Source: CAD feature listing. Evaluate the final solid. Frame: model axes, mm. A direction names the side the tool comes from. Give positions to 0.01 mm unless a question says otherwise; leave off trailing zeros. Loops run counter-clockwise (first coordinate to the right, second up) from the corner with the lowest first, then second, coordinate; pieces in that order, holes last.
from build123d import *

# Parameters (mm, degrees)
SKETCH1_R               = 25
BOSS_EXTRUDE1_DEPTH     = 10
SKETCH2_R               = 17.5
BOSS_EXTRUDE2_DEPTH     = 18
BOSS_EXTRUDE3_DEPTH     = 28
BOSS_EXTRUDE6_DEPTH     = 12
SKETCH5_W               = 12
SKETCH5_H               = 30
CUT_EXTRUDE3_DEPTH      = 35.5
CUT_EXTRUDE3_DEPTH_BACK = 35.5


with BuildPart() as part:
    # Sketch1 → Boss-Extrude1 (new body)
    with BuildSketch(Plane(origin=(0, 0, 0), x_dir=(1, 0, 0), z_dir=(0, 1, 0))):
        Circle(SKETCH1_R)
    extrude(amount=BOSS_EXTRUDE1_DEPTH)

    # Sketch2 → Boss-Extrude2 (add)
    with BuildSketch(Plane(origin=(0, 10, 0), x_dir=(1, 0, 0), z_dir=(0, 1, 0))):
        Circle(SKETCH2_R)
    extrude(amount=BOSS_EXTRUDE2_DEPTH)

    # Sketch3 → Boss-Extrude3 (add)
    with BuildSketch(Plane(origin=(0, 28, 0), x_dir=(1, 0, 0), z_dir=(0, 1, 0))):
        with BuildLine():
            Line((-15.564382416, -8), (15.564382416, -8))
            ThreePointArc((15.564382416, -8), (17.5, 0), (15.564382416, 8))
            Line((15.564382416, 8), (-15.564382416, 8))
            ThreePointArc((-15.564382416, 8), (-17.5, 0), (-15.564382416, -8))
        make_face()
    extrude(amount=BOSS_EXTRUDE3_DEPTH)

    # Sketch4 → Boss-Extrude6 (add, symmetric)
    with BuildSketch(Plane(origin=(0, 0, 0), x_dir=(0, 0, -1), z_dir=(1, 0, 0))):
        Polygon((34.5, 0), (34.5, 7), (25, 28), (-25, 28), (-34.5, 7), (-34.5, 0), align=None)
    extrude(amount=BOSS_EXTRUDE6_DEPTH, both=True)

    # Sketch5 → Cut-Extrude3 (cut, two sides)
    with BuildSketch(Plane.XY) as cut_extrude3_sk:
        with Locations((0, 29)):
            Rectangle(SKETCH5_W, SKETCH5_H)
    extrude(amount=CUT_EXTRUDE3_DEPTH, mode=Mode.SUBTRACT)
    extrude(cut_extrude3_sk.sketch, amount=-CUT_EXTRUDE3_DEPTH_BACK, mode=Mode.SUBTRACT)


solid = part.part
1) Cut plane C-C (z = 24). Return loops of the section in (x, y).
Checks:
outline: (-12, 0) - (12, 0) - (12, 28) - (6, 28) - (6, 14) - (-6, 14) - (-6, 28) - (-12, 28) - close
2) Cut plane D-D (y = 4). Return loops of the section in (x, z).
Checks:
outline: (-12, -34.5) - (12, -34.5) - (12, -21.93) arc R25 ccw to (12, 21.93) - (12, 34.5) - (-12, 34.5) - (-12, 21.93) arc R25 ccw to (-12, -21.93) - close
3) Contact query for flat-ended pins moving along their axis: P1, Ø5, axis at x = -19.5, y = 11.5, coming from the +Z side; P2, Ø6.5, axis at y = 15.5, z = -21.5, coming from the -X side; P3, Ø22.5, axis at x = -1.5, y = 43, coming from the -Z side. Output: stop coordinate, or through.
Checks:
P1: stops at z = 17.85
P2: stops at x = -12
P3: stops at z = -8
4) Cut plane B-B (y = 36). Return loops of the section in (x, z).
Checks:
outline: (-15.56, -8) - (-6, -8) - (-6, 8) - (-15.56, 8) arc R17.5 ccw to start; (6, -8) - (15.56, -8) arc R17.5 ccw to (15.56, 8) - (6, 8) - close
5) Reachability of faces 4 (the flat face through (10, 28, -17)), 5 (the flat face through (-10, 28, 16)), 6 (the cylindrical face through (-17.5, 27.6, -0.2)), 7 (the flat face through (18, 10, 0)) from +Z, -Z, +X, -X, +Y, -Y: full face, straight path, thin tool, end or side. Return the list, or none.
Checks:
face 4: -Z, +X, -X, +Y
face 5: +Z, +X, -X, +Y
face 6: -X, +Y
face 7: +X, +Y
6) Pull-direction query (Y, two-part tool) for faces 1 (the flat face through (0, 14, 0)), 2 (the flat face through (-12, 14, 24)), 3 (the flat face through (0.168, 12.98, 31.795)); classes: released by +Y, released by -Y, zero draft, split by the parting line, or undercut.
Checks:
face 1: undercut
face 2: zero draft
face 3: released by +Y
7) Ray query, probe 1 along Y at (x, z) = (4, -1); probe 2 along X at (y, z) = (15, -25.5); probe 3 along Z at (x, y) = (-21.5, 5.5). Return the intervals inside material, ascending.
Checks:
probe 1: y = 0 to 14, 44 to 56
probe 2: x = -12 to -6, 6 to 12
probe 3: z = -12.76 to 12.76
8) Cut plane A-A (x = 1). Return loops of the section in (y, z).
Checks:
outline: (0, -34.5) - (7, -34.5) - (14, -31.33) - (14, 31.33) - (7, 34.5) - (0, 34.5) - close; (44, -8) - (56, -8) - (56, 8) - (44, 8) - close
